Design review of the part built by this model. Coordinates are the model's own, in mm. Face numbers are marked on the shaded views. A direction names the side the tool comes from. Round coordinates to 2 decimals unless told otherwise and drop trailing zeros. Write each loop counter-clockwise with the first axis right and the second up, starting at its lowest first coordinate (ties: lowest second). Pieces come first, ordered by that corner, then holes.
from build123d import *

# Parameters (mm, degrees)
SKETCH1_R           = 25.4
SKETCH1_R_2         = 12.7
BOSS_EXTRUDE1_DEPTH = 20
SKETCH2_R           = 2
CUT_EXTRUDE1_DEPTH  = 30
CUT_EXTRUDE2_START  = -3.5687
SKETCH3_R           = 19.84375
SKETCH3_R_2         = 12.7
CUT_EXTRUDE2_DEPTH  = 3.5687
SKETCH5_R           = 1.65
CUT_EXTRUDE4_DEPTH  = 31.7
SKETCH6_W           = 56.4
SKETCH6_H           = 56.4
SKETCH6_R           = 12.7
SKETCH6_R_2         = 2.5
BOSS_EXTRUDE2_DEPTH = 5
SKETCH7_R           = 19.5
CUT_EXTRUDE5_DEPTH  = 2


with BuildPart() as part:
    # Sketch1 → Boss-Extrude1 (new body)
    with BuildSketch(Plane.XY):
        Circle(SKETCH1_R)
        Circle(SKETCH1_R_2, mode=Mode.SUBTRACT)
    extrude(amount=BOSS_EXTRUDE1_DEPTH)

    # Sketch2 → Cut-Extrude1 (cut, symmetric)
    with BuildSketch(Plane(origin=(0, 0, 0), x_dir=(0, 0, -1), z_dir=(1, 0, 0))):
        with Locations((-10, 0)):
            Circle(SKETCH2_R)
    extrude(amount=CUT_EXTRUDE1_DEPTH, both=True, mode=Mode.SUBTRACT)

    # Sketch3 → Cut-Extrude2 (cut)
    with BuildSketch(Plane.XY.offset(20).offset(CUT_EXTRUDE2_START)):
        Circle(SKETCH3_R)
        Circle(SKETCH3_R_2, mode=Mode.SUBTRACT)
    extrude(amount=CUT_EXTRUDE2_DEPTH, mode=Mode.SUBTRACT)

    # Sketch5 → Cut-Extrude4 (cut, symmetric)
    with BuildSketch(Plane(origin=(0, 0, 0), x_dir=(1, 0, 0), z_dir=(0, 1, 0))):
        with Locations(Location((0, -10, 0), (0, 0, 270))):
            Circle(SKETCH5_R)
    extrude(amount=CUT_EXTRUDE4_DEPTH, both=True, mode=Mode.SUBTRACT)

    # Sketch6 → Boss-Extrude2 (add)
    with BuildSketch(Plane(origin=(0, 0, 0), x_dir=(-1, 0, 0), z_dir=(0, 0, -1))):
        Rectangle(SKETCH6_W, SKETCH6_H)
        with Locations(Location((0, 0, 0), (0, 0, 180))):
            Circle(SKETCH6_R, mode=Mode.SUBTRACT)
        with Locations((-23.55, 23.55)):
            Circle(SKETCH6_R_2, mode=Mode.SUBTRACT)
        with Locations((23.55, 23.55)):
            Circle(SKETCH6_R_2, mode=Mode.SUBTRACT)
        with Locations((23.55, -23.55)):
            Circle(SKETCH6_R_2, mode=Mode.SUBTRACT)
        with Locations((-23.55, -23.55)):
            Circle(SKETCH6_R_2, mode=Mode.SUBTRACT)
    extrude(amount=-BOSS_EXTRUDE2_DEPTH)

    # Sketch7 → Cut-Extrude5 (cut)
    with BuildSketch(Plane(origin=(0, 0, 0), x_dir=(-1, 0, 0), z_dir=(0, 0, -1))):
        Circle(SKETCH7_R)
    extrude(amount=-CUT_EXTRUDE5_DEPTH, mode=Mode.SUBTRACT)


solid = part.part
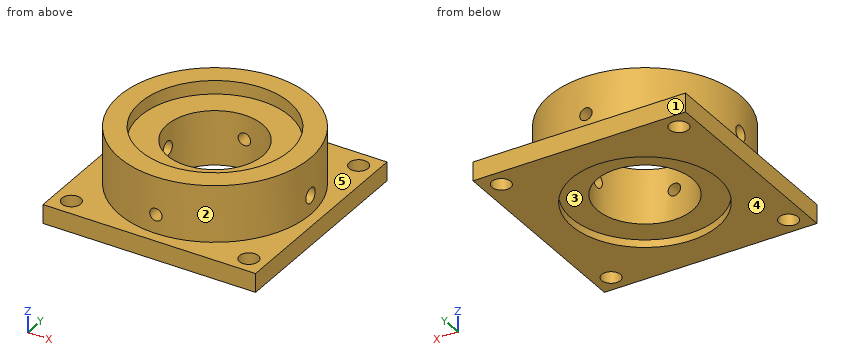
1) Add section C-C on x = -23.55. State the section outline as (y, z) points, and give its area (3 significant figures).
2) The part is to be moulded in two halves that separate along X. For the marked faces 1, 2 and 3, say which applies: pulls with the +X half, pulls with the -X half, needs draft (parallel to the pull), parting line crosses it, or undercut.
3) Add section D-D on z = 3.5. State the section outline as (x, y) points, and give its area (3 significant figures).
4) Add section A-A on x = 0. State the section outline as (y, z) points, and give its area (3 significant figures).
5) For the marked faces 4 and 5, list the 3-axis set-ups (+Z, -Z, +X, -X, +Y, -Y) from which the entire face can be reached by the end or side of a thin tool; tool diameter is ignored.
6) For line 1 along Y through (x, z) = (23.55, 2.8); line 2 along Y through (x, z) = (0, 1.1); line 3 along Y through (x, z) = (0, 19.25), list the stretches that pass through material, from the lowest coordinate up.
7) For P1, Ø4, axis at y = 5.5, z = 10, coming from the +X side; P2, Ø3, axis at x = -8, y = -17, coming from the -Z side; P3, Ø23, axis at x = 0, y = 0, coming from the -Z side; P4, Ø1, axis at x = 12.5, z = 16, coming from the +Y side, all flat-tipped, find the tip position at first contact; note any pin that passes through.
8) Add section B-B on y = 22. State the section outline as (x, z) points, and give its area (3 significant figures).
Computed:
1. outline: (-28.2, 0) - (-26.05, 0) - (-26.05, 5) - (-28.2, 5) - close; (-21.05, 0) - (21.05, 0) - (21.05, 5) - (9.52, 5) - (9.52, 20) - (-9.52, 20) - (-9.52, 5) - (-21.05, 5) - close; (26.05, 0) - (28.2, 0) - (28.2, 5) - (26.05, 5) - close; hole circle Ø4 at (0, 10)
1. area: 505 mm2
2. face 1: needs draft
2. face 2: parting line crosses it
2. face 3: undercut
3. outline: (-28.2, -28.2) - (28.2, -28.2) - (28.2, 28.2) - (-28.2, 28.2) - close; hole circle Ø5 at (-23.55, -23.55); hole circle Ø5 at (-23.55, 23.55); hole circle Ø25.4 at (0, 0); hole circle Ø5 at (23.55, -23.55); hole circle Ø5 at (23.55, 23.55)
3. area: 2,600 mm2
4. outline: (-28.2, 0) - (-19.5, 0) - (-19.5, 2) - (-12.7, 2) - (-12.7, 8.35) - (-25.4, 8.35) - (-25.4, 5) - (-28.2, 5) - close; (-25.4, 11.65) - (-12.7, 11.65) - (-12.7, 16.43) - (-19.84, 16.43) - (-19.84, 20) - (-25.4, 20) - close; (12.7, 2) - (19.5, 2) - (19.5, 0) - (28.2, 0) - (28.2, 5) - (25.4, 5) - (25.4, 8.35) - (12.7, 8.35) - close; (12.7, 11.65) - (25.4, 11.65) - (25.4, 20) - (19.84, 20) - (19.84, 16.43) - (12.7, 16.43) - close
4. area: 374 mm2
5. face 4: -Z, +X, -X, +Y, -Y
5. face 5: +Z
6. line 1: y = -28.2 to -26.05, -21.05 to 21.05, 26.05 to 28.2
6. line 2: y = -28.2 to -19.5, 19.5 to 28.2
6. line 3: y = -25.4 to -19.84, 19.84 to 25.4
7. P1: stops at x = 25.16
7. P2: stops at z = 0
7. P3: passes through
7. P4: stops at y = 22.39
8. outline: (-28.2, 0) - (-25.51, 0) - (-25.51, 5) - (-28.2, 5) - close; (-21.59, 0) - (21.59, 0) - (21.59, 5) - (12.69, 5) - (12.69, 20) - (-12.69, 20) - (-12.69, 5) - (-21.59, 5) - close; (25.51, 0) - (28.2, 0) - (28.2, 5) - (25.51, 5) - close; hole circle Ø3.3 at (0, 10)
8. area: 615 mm2
